Read the model definition and answer for the solid it produces. Units are mm, in the model's axes. A direction names the side the tool comes from. Coordinates: 2 decimals unless noted, no trailing zeros. Write each loop counter-clockwise with the first axis right and the second up, starting at its lowest first coordinate (ties: lowest second). Pieces come first, ordered by that corner, then holes.
1) The part is cut by section D-D (y = -40.5). Determine the outline of the cut face in (x, z), then the cut area to 3 significant figures.
2) Find the intervals of material crossed by line 1 (X direction, y = -34.5, z = 44.5); line 2 (Z direction, x = 48.5, y = -33); line 3 (X direction, y = -24.5, z = 3), in increasing order.
3) The part is cut by section A-A (y = -36). Determine the outline of the cut face in (x, z).
4) The part is cut by section C-C (z = 31.5). Determine the outline of the cut face in (x, y), then the cut area to 3 significant figures.
5) Each of these flat-tipped pins is pushed along its axis until it touches: pin 1 Ø3 at (x, z) = (37, 34.5) entering from -Y; pin 2 Ø10 at (x, z) = (34, 28.5) entering from +Y; pin 3 Ø12 at (x, z) = (53, 11.5) entering from -Y. Where does it stop, or does it pass through?
6) Which of the six approach directions +Z, -Z, +X, -X, +Y, -Y give full straight-line access (tool end or side, diameter ignored) to faces 1 (the face through (29.22, -26.474, -2.465)), 2 (the face through (43.6, -22.57, -2.46)), 3 (the face through (55.52, -31.25, -2.46))?
7) The part is cut by section B-B (x = 46). Determine the outline of the cut face in (y, z).
8) Determine the mould class of faces 4 (the face through (49.242, -22.132, -2.465)), 5 (the face through (28, -32, -5)), 6 (the face through (27.287, -37.375, -2.465)) for opening direction X: +X half, -X half, draft (parallel to the pull), parting line (faces both ways), or undercut.
from build123d import *

# Parameters (mm, degrees)
F0_R     = 16
F1_DEPTH = 50
F3_DEPTH = 5


# Not quite as in the source:
# - after a boolean that leaves OpenCascade's solid faulty, fix() repairs it


with BuildPart() as f1:
    # F0 (on Top) → F1 (new body)
    with BuildSketch(Plane.XY):
        with Locations((41.4022505283, -34.313749522)):
            Circle(F0_R)
    extrude(amount=F1_DEPTH)

    # F2 (on face) → F3 (join)
    with BuildSketch(Plane(origin=(0, 0, 0), x_dir=(1, 0, 0), z_dir=(0, 0, -1))):
        Polygon((57.0387140238, 30.9224357125), (54.8569208916, 42.9723779016), (52.2755180634, 41.3111400427), (54.0387140238, 31.573090602), align=None)
        with BuildLine():
            ThreePointArc((57.0387140238, 30.9224357125), (57.3111068029, 32.6083779976), (57.4022505283, 34.313749522))
            ThreePointArc((57.4022505283, 34.313749522), (56.7527346544, 38.8262473994), (54.8569208916, 42.9723779016))
            Line((54.8569208916, 42.9723779016), (57.0387140238, 30.9224357125))
        make_face()
        Polygon((38.0109367189, 18.6772860265), (50.060878908, 20.8590791587), (48.399641049, 23.4404819869), (38.6615916084, 21.6772860265), align=None)
        with BuildLine():
            ThreePointArc((38.0109367189, 18.6772860265), (44.252900632, 18.5697413288), (50.060878908, 20.8590791587))
            Line((50.060878908, 20.8590791587), (38.0109367189, 18.6772860265))
        make_face()
        Polygon((28.7657870328, 37.0544084419), (25.7657870328, 37.7050633314), (27.9475801651, 25.6551211423), (30.5289829933, 27.3163590013), align=None)
        with BuildLine():
            Line((27.9475801651, 25.6551211423), (25.7657870328, 37.7050633314))
            ThreePointArc((25.7657870328, 37.7050633314), (25.6582423352, 31.4630994183), (27.9475801651, 25.6551211423))
        make_face()
        Polygon((44.1429094483, 46.9502130175), (44.7935643378, 49.9502130175), (32.7436221487, 47.7684198852), (34.4048600077, 45.187017057), align=None)
        with BuildLine():
            Line((32.7436221487, 47.7684198852), (44.7935643378, 49.9502130175))
            ThreePointArc((44.7935643378, 49.9502130175), (38.5516004247, 50.0577577151), (32.7436221487, 47.7684198852))
        make_face()
    extrude(amount=F3_DEPTH)

    add(f1.part.fix(), mode=Mode.REPLACE)


solid = f1.part
Reported:
1. outline: (26.65, 0) - (52.42, 0) - (52.42, -5) - (56.16, -5) - (56.16, 50) - (26.65, 50) - close
1. area: 1,490 mm2
2. line 1: x = 25.4 to 57.4
2. line 2: z = 0 to 50
2. line 3: x = 28.77 to 54.04
3. outline: (25.49, -5) - (28.96, -5) - (28.96, 0) - (53.24, 0) - (53.24, -5) - (57.31, -5) - (57.31, 50) - (25.49, 50) - close
4. outline: circle Ø32 at (41.4, -34.31)
4. area: 804 mm2
5. pin 1: stops at y = -50.05
5. pin 2: stops at y = -18.5
5. pin 3: stops at y = -49.3
6. face 1: -Z, +X, +Y
6. face 2: -Z, -X
6. face 3: -Z, +Y
7. outline: (-49.64, 0) - (-23.01, 0) - (-23.01, -5) - (-18.99, -5) - (-18.99, 50) - (-49.64, 50) - close
8. face 4: +X half
8. face 5: draft
8. face 6: undercut
